```python
from build123d import *

# Parameters (mm, degrees)
SZKIC1_W                    = 60
SZKIC1_H                    = 60
DODANIE_WYCI_GNI_CIE1_DEPTH = 200
SKORUPA1_T                  = -3
SZKIC2_W                    = 5
SZKIC2_H                    = 5
SZKIC2_R                    = 1
DODANIE_WYCI_GNI_CIE2_DEPTH = 57
SZKIC4_W                    = 5
SZKIC4_H                    = 5
SZKIC4_R                    = 1
DODANIE_WYCI_GNI_CIE3_DEPTH = 57
SZKIC5_W                    = 5
SZKIC5_H                    = 5
SZKIC5_R                    = 1
DODANIE_WYCI_GNI_CIE4_DEPTH = 57
SZKIC6_W                    = 5
SZKIC6_H                    = 5
SZKIC6_R                    = 1
DODANIE_WYCI_GNI_CIE6_DEPTH = 57
SZKIC9_R                    = 12.625
WYTNIJ_WYCI_GNI_CIE1_DEPTH  = 3
SZKIC10_W                   = 45.55
SZKIC10_H                   = 7.6
DODANIE_WYCI_GNI_CIE7_DEPTH = 32.45
SZKIC13_R                   = 1.5
WYTNIJ_WYCI_GNI_CIE4_DEPTH  = 5
SZKIC14_R                   = 1.5
WYTNIJ_WYCI_GNI_CIE5_DEPTH  = 5
WYTNIJ_WYCI_GNI_CIE7_DEPTH  = 10


with BuildPart() as part:
    # Szkic1 → Dodanie-wyciągnięcie1 (new body)
    with BuildSketch(Plane(origin=(0, 0, 0), x_dir=(1, 0, 0), z_dir=(0, 1, 0))):
        with Locations((30, 30)):
            Rectangle(SZKIC1_W, SZKIC1_H)
    extrude(amount=DODANIE_WYCI_GNI_CIE1_DEPTH)

    # Skorupa1
    skorupa1_openings = [part.faces().sort_by_distance(p)[0] for p in [
        (30, 100, 0),
    ]]
    offset(amount=SKORUPA1_T, openings=skorupa1_openings, kind=Kind.INTERSECTION)

    # Szkic2 → Dodanie-wyciągnięcie2 (add)
    with BuildSketch(Plane.XY.offset(-57)):
        with Locations((5.5, 194.5)):
            Rectangle(SZKIC2_W, SZKIC2_H)
        with Locations(Location((5.5, 194.5, 0), (0, 0, 180))):
            Circle(SZKIC2_R, mode=Mode.SUBTRACT)
    extrude(amount=DODANIE_WYCI_GNI_CIE2_DEPTH)

    # Szkic4 → Dodanie-wyciągnięcie3 (add)
    with BuildSketch(Plane.XY):
        with Locations((54.5, 194.5)):
            Rectangle(SZKIC4_W, SZKIC4_H)
        with Locations((54.5, 194.5)):
            Circle(SZKIC4_R, mode=Mode.SUBTRACT)
    extrude(amount=-DODANIE_WYCI_GNI_CIE3_DEPTH)

    # Szkic5 → Dodanie-wyciągnięcie4 (add)
    with BuildSketch(Plane.XY.offset(-57)):
        with Locations((5.5, 5.5)):
            Rectangle(SZKIC5_W, SZKIC5_H)
        with Locations(Location((5.5, 5.5, 0), (0, 0, 180))):
            Circle(SZKIC5_R, mode=Mode.SUBTRACT)
    extrude(amount=DODANIE_WYCI_GNI_CIE4_DEPTH)

    # Szkic6 → Dodanie-wyciągnięcie6 (add)
    with BuildSketch(Plane.XY.offset(-57)):
        with Locations((54.5, 5.5)):
            Rectangle(SZKIC6_W, SZKIC6_H)
        with Locations(Location((54.5, 5.5, 0), (0, 0, 180))):
            Circle(SZKIC6_R, mode=Mode.SUBTRACT)
    extrude(amount=DODANIE_WYCI_GNI_CIE6_DEPTH)

    # Szkic9 → Wytnij-wyciągnięcie1 (cut)
    with BuildSketch(Plane(origin=(60, 0, 0), x_dir=(0, 0, -1), z_dir=(1, 0, 0))):
        with Locations((34.18, 159.82)):
            Circle(SZKIC9_R)
    extrude(amount=-WYTNIJ_WYCI_GNI_CIE1_DEPTH, mode=Mode.SUBTRACT)

    # Szkic10 → Dodanie-wyciągnięcie7 (add)
    with BuildSketch(Plane(origin=(3, 0, 0), x_dir=(0, 0, -1), z_dir=(1, 0, 0))):
        with Locations((34.225, 173.56)):
            Rectangle(SZKIC10_W, SZKIC10_H)
        with Locations((34.225, 124.96)):
            Rectangle(SZKIC10_W, SZKIC10_H)
    extrude(amount=DODANIE_WYCI_GNI_CIE7_DEPTH)

    # Szkic13 → Wytnij-wyciągnięcie4 (cut)
    with BuildSketch(Plane(origin=(35.45, 0, 0), x_dir=(0, 0, -1), z_dir=(1, 0, 0))):
        with Locations((25.1, 174.36)):
            Circle(SZKIC13_R)
        with Locations((15.45, 174.36)):
            Circle(SZKIC13_R)
    extrude(amount=-WYTNIJ_WYCI_GNI_CIE4_DEPTH, mode=Mode.SUBTRACT)

    # Szkic14 → Wytnij-wyciągnięcie5 (cut)
    with BuildSketch(Plane(origin=(35.45, 0, 0), x_dir=(0, 0, -1), z_dir=(1, 0, 0))):
        with Locations((25.6, 124.16)):
            Circle(SZKIC14_R)
        with Locations((15.45, 124.16)):
            Circle(SZKIC14_R)
    extrude(amount=-WYTNIJ_WYCI_GNI_CIE5_DEPTH, mode=Mode.SUBTRACT)

    # Szkic15 → Wytnij-wyciągnięcie7 (cut)
    with BuildSketch(Plane(origin=(0, 177.36, 0), x_dir=(1, 0, 0), z_dir=(0, 1, 0))):
        Polygon((17.95, 11.45), (3, 11.45), (3, 26.45), align=None)
    extrude(amount=-WYTNIJ_WYCI_GNI_CIE7_DEPTH, mode=Mode.SUBTRACT)


solid = part.part
```
Work out the finished part from the listing and answer in its coordinate system (mm). A direction names the side the tool comes from. Give positions to 0.01 mm unless a question says otherwise; leave off trailing zeros. Order: outer loops, then holes, each group sorted by start corner. A loop starts at its lowest first (then second) coordinate and runs counter-clockwise, first axis right, second up.
1. Section C-C, the plane y = 15 is taken. Determine the outline of the cut face in (x, z).
Result sheet:
outline: (0, -60) - (60, -60) - (60, 0) - (57, 0) - (57, -57) - (3, -57) - (3, 0) - (0, 0) - close
2. Section B-B, the plane z = -34.18 is taken. Give the number of separate pieces and of enclosed holes in the cut face, and give its area (3 significant figures).
Result sheet:
separate pieces: 1
enclosed holes: 4
area: 2,030 mm2
3. Section D-D, the plane y = 165.5 is taken. Determine the outline of the cut face in (x, z), and give its area (3 significant figures).
Result sheet:
outline: (0, -60) - (60, -60) - (60, -45.46) - (57, -45.46) - (57, -57) - (3, -57) - (3, 0) - (0, 0) - close; (57, -22.9) - (60, -22.9) - (60, 0) - (57, 0) - close
area: 454 mm2
4. Each of these flat-tipped pins is pushed along its axis until it touches: P1, Ø1.8, axis at x = 54.5, y = 5.5, coming from the +Z side; P2, Ø4, axis at x = 12, y = 125.5, coming from the +Z side. Where does it stop, or does it pass through?
Result sheet:
P1: stops at z = -57
P2: stops at z = -11.45
5. For faces 1 (the flat face through (52, 194, -28)), 2 (the flat face through (0, 99, -30)), determine the directions among +Z, -Z, +X, -X, +Y, -Y from which every point of the face is accessible in a straight line to the end or side of a thin tool.
Result sheet:
face 1: +Z
face 2: +Z, -Z, -X, +Y, -Y
6. The mould has two halves that part along Z. Classify faces 3 (the flat face through (60, 99, -30)), 4 (the cylindrical face through (58.52, 148.62, -40.01)), 5 (the flat face through (19, 125, -11.45)): released by +Z, released by -Z, zero draft, split by the parting line, or undercut.
Result sheet:
face 3: zero draft
face 4: undercut
face 5: released by +Z
7. Section A-A, the plane x = 33.5 is taken. Determine the outline of the cut face in (y, z), and give its area (3 significant figures).
Result sheet:
outline: (0, -60) - (200, -60) - (200, 0) - (197, 0) - (197, -57) - (177.36, -57) - (177.36, -11.45) - (169.76, -11.45) - (169.76, -57) - (128.76, -57) - (128.76, -11.45) - (121.16, -11.45) - (121.16, -57) - (3, -57) - (3, 0) - (0, 0) - close; hole circle Ø3 at (124.16, -25.6); hole circle Ø3 at (124.16, -15.45); hole circle Ø3 at (174.36, -25.1); hole circle Ø3 at (174.36, -15.45)
area: 1,610 mm2
8. Straight lines are drawn through the part: L1, parallel to Z at x = 32, y = 174; L2, parallel to X at y = 194.5, z = -43.5; L3, parallel to Y at x = 21, z = -27. For each, find the intervals that lie inside material, in ascending order.
Result sheet:
L1: z = -60 to -26.56, -23.64 to -16.91, -13.99 to -11.45
L2: x = 0 to 4.5, 6.5 to 8, 52 to 53.5, 55.5 to 60
L3: y = 0 to 3, 121.16 to 128.76, 169.76 to 177.36, 197 to 200
